from build123d import *

# Parameters (mm, degrees)
SKETCH_1_W          = 10
SKETCH_1_H          = 20
SKETCH_1_R          = 1.75
EXTRUDE_1_DEPTH     = 2.5
SKETCH_2_W          = 1
SKETCH_2_H          = 6
CUT_EXTRUDE_1_DEPTH = 0.8


with BuildPart() as part:
    # Эскиз1 → Бобышка-Вытянуть1 (new body)
    with BuildSketch(Plane.XY):
        with Locations((5, 10)):
            Rectangle(SKETCH_1_W, SKETCH_1_H)
        with Locations((5, 17)):
            Circle(SKETCH_1_R, mode=Mode.SUBTRACT)
        with Locations((5, 3)):
            Circle(SKETCH_1_R, mode=Mode.SUBTRACT)
    extrude(amount=EXTRUDE_1_DEPTH)

    # Эскиз2 → Вырез-Вытянуть1 (cut)
    with BuildSketch(Plane.XY.offset(2.5)):
        with Locations((0.5, 10)):
            Rectangle(SKETCH_2_W, SKETCH_2_H)
        with Locations((2.5, 10)):
            Rectangle(SKETCH_2_W, SKETCH_2_H)
        with Locations((4.5, 10)):
            Rectangle(SKETCH_2_W, SKETCH_2_H)
        with Locations((6.5, 10)):
            Rectangle(SKETCH_2_W, SKETCH_2_H)
        with Locations((8.5, 10)):
            Rectangle(SKETCH_2_W, SKETCH_2_H)
    extrude(amount=-CUT_EXTRUDE_1_DEPTH, mode=Mode.SUBTRACT)


solid = part.part
Work out the finished part from the listing and answer in its coordinate system (mm). A direction names the side the tool comes from. Round coordinates to 2 decimals unless told otherwise and drop trailing zeros. Write each loop counter-clockwise with the first axis right and the second up, starting at its lowest first coordinate (ties: lowest second). Pieces come first, ordered by that corner, then holes.
1) A cutting plane is placed at A-A (y = 3). Give the vertices of the cut face in (x, z), plus the area to 4 significant figures.
2) A cutting plane is placed at D-D (y = 9.5). Give the vertices of the cut face in (x, z), plus the area to 3 significant figures.
3) A cutting plane is placed at B-B (z = 2.05). Give the vertices of the cut face in (x, y), plus the area to 3 significant figures.
4) A tool of negligible diameter and unlimited length cuts with its end or side. For faces 4 (the flat face through (4.5, 10, 1.7)), 5 (the flat face through (0.5, 10, 1.7)), 6 (the flat face through (5, 20, 1)), from which of +Z, -Z, +X, -X, +Y, -Y can it reach the whole face along a straight path? Write none if from no direction.
5) Straight lines are drawn through the part: line 1 (Y direction, x = 5, z = 0.9); line 2 (X direction, y = 8.25, z = 2.05); line 3 (Y direction, x = 6, z = 1.05). For each, find the intervals that lie inside material, in ascending order.
6) Given pin 1 Ø1.5 at (x, y) = (2.5, 11.5) entering from +Z, flat-ended and moving along its own axis, determine where the tip first touches the part or whether it passes through.
7) The mould has two halves that part along Y. Classify faces 1 (the flat face through (10, 10, 1)), 2 (the flat face through (8.5, 10, 1.7)), 3 (the flat face through (5, 0, 1)): pulls with the +Y half, pulls with the -Y half, needs draft (parallel to the pull), parting line crosses it, or undercut.
8) A cutting plane is placed at C-C (x = 6.25). Give the vertices of the cut face in (y, z).
Completed:
1. outline: (0, 0) - (3.25, 0) - (3.25, 2.5) - (0, 2.5) - close; (6.75, 0) - (10, 0) - (10, 2.5) - (6.75, 2.5) - close
1. area: 16.25 mm2
2. outline: (0, 0) - (10, 0) - (10, 2.5) - (9, 2.5) - (9, 1.7) - (8, 1.7) - (8, 2.5) - (7, 2.5) - (7, 1.7) - (6, 1.7) - (6, 2.5) - (5, 2.5) - (5, 1.7) - (4, 1.7) - (4, 2.5) - (3, 2.5) - (3, 1.7) - (2, 1.7) - (2, 2.5) - (1, 2.5) - (1, 1.7) - (0, 1.7) - close
2. area: 21.0 mm2
3. outline: (0, 0) - (10, 0) - (10, 20) - (0, 20) - (0, 13) - (1, 13) - (1, 7) - (0, 7) - close; hole (2, 7) - (3, 7) - (3, 13) - (2, 13) - close; hole circle Ø3.5 at (5, 3); hole circle Ø3.5 at (5, 17); hole (4, 7) - (5, 7) - (5, 13) - (4, 13) - close; hole (6, 7) - (7, 7) - (7, 13) - (6, 13) - close; hole (8, 7) - (9, 7) - (9, 13) - (8, 13) - close
3. area: 151 mm2
4. face 4: +Z
4. face 5: +Z, -X
4. face 6: +Z, -Z, +X, -X, +Y
5. line 1: y = 0 to 1.25, 4.75 to 15.25, 18.75 to 20
5. line 2: x = 1 to 2, 3 to 4, 5 to 6, 7 to 8, 9 to 10
5. line 3: y = 0 to 1.56, 4.44 to 15.56, 18.44 to 20
6. pin 1: stops at z = 2.5
7. face 1: needs draft
7. face 2: undercut
7. face 3: pulls with the -Y half
8. outline: (0, 0) - (1.78, 0) - (1.78, 2.5) - (0, 2.5) - close; (4.22, 0) - (15.78, 0) - (15.78, 2.5) - (13, 2.5) - (13, 1.7) - (7, 1.7) - (7, 2.5) - (4.22, 2.5) - close; (18.22, 0) - (20, 0) - (20, 2.5) - (18.22, 2.5) - close
